Print and shaded views of the part. All mm, measured from the part's lowest x, y and z. A direction names the side the tool comes from. Give positions to 0.01 mm unless a question says otherwise; leave off trailing zeros. Order: outer loops, then holes, each group sorted by start corner. A loop starts at its lowest first (then second) coordinate and runs counter-clockwise, first axis right, second up. Notation, with made-up numbers: (55, 18) -> (67, 18) arc R25 ccw to (67, 56) -> close; hole circle Ø6 at (-1.5, 27.5). An arc over 180 degrees is marked (long way). One line per question, with ' | ' between items. Start each with the question number.
(1) Pin check, flat tips, straight feed: pin 1 Ø9.5 at (y, z) = (9, 8.5) entering from -X; pin 2 Ø4 at (x, z) = (35, 10) entering from -Y; pin 3 Ø7 at (x, z) = (5, 10) entering from +Y. Stop position of each tip, or through.
(2) Cut at D-D (x = 20). Give the cut face in (y, z), then the cut area to 3 significant figures.
(3) Cut at A-A (x = 5). Give the cut face in (y, z), then the cut area to 3 significant figures.
(4) Cut at C-C (z = 18.25). Give the cut face in (x, y).
(5) Cut at B-B (z = 10.75). Give the cut face in (x, y), then the cut area to 3 significant figures.
(6) Drill centre lines: L1, parallel to Z at x = 5, y = 1.2; L2, parallel to Z at x = 27.5, y = 22.25; L3, parallel to Y at x = 24, z = 22.5. Where is each one in solid material? Low to high. Write a range as from..to.
(7) Which spindle directions (+Z, -Z, +X, -X, +Y, -Y) get a long thin tool onto all of the face, cutting with end or side? Do the marked faces 1 and 2. Say none if no direction does.
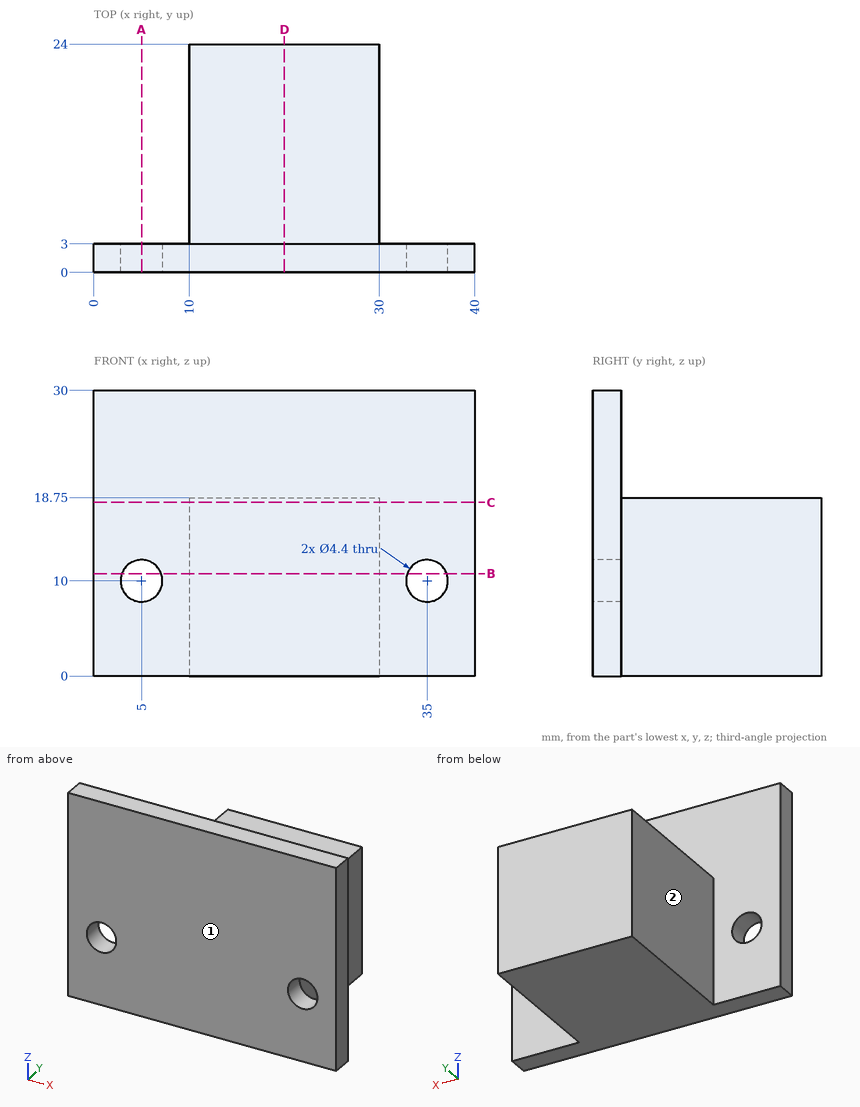
Result set:
1) pin 1: stops at x = 10 | pin 2: passes through | pin 3: stops at y = 3
2) outline: (0, 0) -> (24, 0) -> (24, 18.75) -> (3, 18.75) -> (3, 30) -> (0, 30) -> close | area: 484 mm2
3) outline: (0, 0) -> (3, 0) -> (3, 7.8) -> (0, 7.8) -> close; (0, 12.2) -> (3, 12.2) -> (3, 30) -> (0, 30) -> close | area: 76.8 mm2
4) outline: (0, 0) -> (40, 0) -> (40, 3) -> (30, 3) -> (30, 24) -> (10, 24) -> (10, 3) -> (0, 3) -> close
5) outline: (0, 0) -> (2.93, 0) -> (2.93, 3) -> (0, 3) -> close; (7.07, 0) -> (32.93, 0) -> (32.93, 3) -> (30, 3) -> (30, 24) -> (10, 24) -> (10, 3) -> (7.07, 3) -> close; (37.07, 0) -> (40, 0) -> (40, 3) -> (37.07, 3) -> close | area: 515 mm2
6) L1: z = 0..7.8, 12.2..30 | L2: z = 0..18.75 | L3: y = 0..3
7) face 1: +Z, -Z, +X, -X, -Y | face 2: +Z, -Z, -X, +Y
